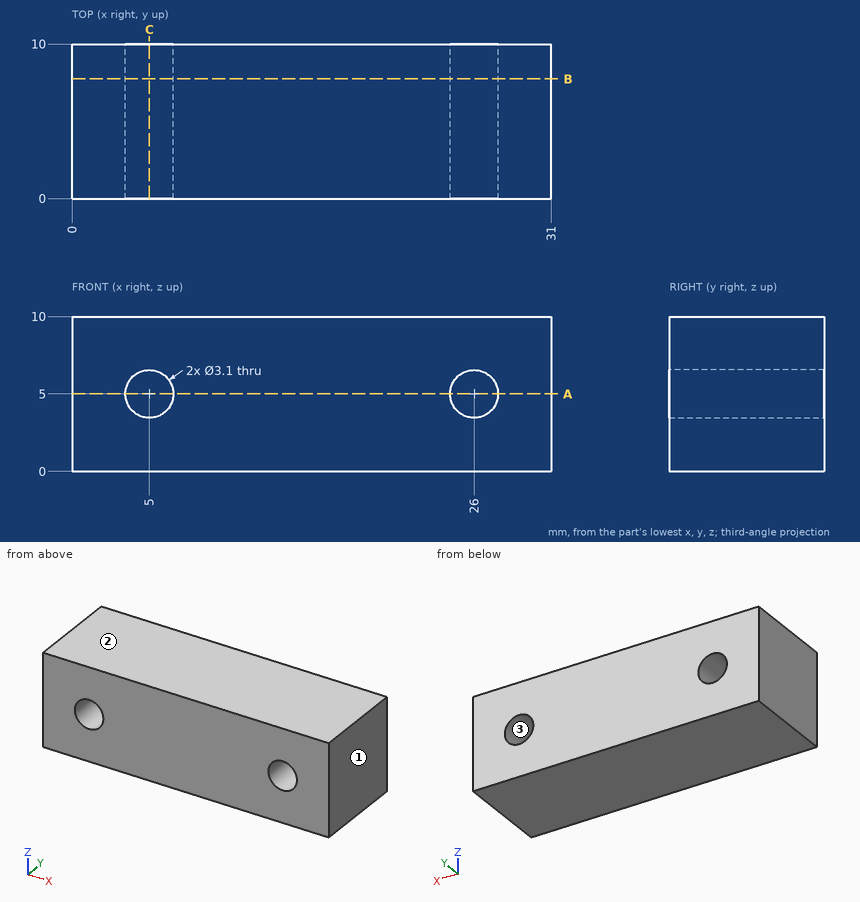
Design review of the part shown in the three views and the two pictorial views. Dimensions are in mm from the part's minimum x, y and z. Coordinates: 2 decimals unless noted, no trailing zeros. Order: outer loops, then holes, each group sorted by start corner. A loop starts at its lowest first (then second) coordinate and runs counter-clockwise, first axis right, second up.
Item 1: The part is to be moulded in two halves that separate along X. For the marked faces 1, 2 and 3, say which applies: pulls with the +X half, pulls with the -X half, needs draft (parallel to the pull), parting line crosses it, or undercut.
Item 2: Take a section at B-B, the plane y = 7.75. Write out the cut boundary in (x, z).
Item 3: For line 1 (X direction, y = 4.5, z = 5); line 2 (Z direction, x = 27, y = 7.75), list the stretches that pass through material, from the lowest coordinate up.
Item 4: Take a section at C-C, the plane x = 5. Write out the cut boundary in (y, z), then the cut area to 3 significant figures.
Item 5: Take a section at A-A, the plane z = 5. Write out the cut boundary in (x, y), then the cut area to 3 significant figures.
Item 6: For pin 1 Ø1 at (y, z) = (4.5, 3.5) entering from -X, flat-tipped, find the tip position at first contact; note if it passes through.
The answers:
1. face 1: pulls with the +X half
1. face 2: needs draft
1. face 3: undercut
2. outline: (0, 0) - (31, 0) - (31, 10) - (0, 10) - close; hole circle Ø3.1 at (5, 5); hole circle Ø3.1 at (26, 5)
3. line 1: x = 0 to 3.45, 6.55 to 24.45, 27.55 to 31
3. line 2: z = 0 to 3.82, 6.18 to 10
4. outline: (0, 0) - (10, 0) - (10, 3.45) - (0, 3.45) - close; (0, 6.55) - (10, 6.55) - (10, 10) - (0, 10) - close
4. area: 69.0 mm2
5. outline: (0, 0) - (3.45, 0) - (3.45, 10) - (0, 10) - close; (6.55, 0) - (24.45, 0) - (24.45, 10) - (6.55, 10) - close; (27.55, 0) - (31, 0) - (31, 10) - (27.55, 10) - close
5. area: 248 mm2
6. pin 1: stops at x = 0
